Could you check a few things on this drawing? It's one solid part, dimensions in mm from its lowest x, y, z. A direction names the side the tool comes from. Coordinates: 2 decimals unless noted, no trailing zeros. Write each loop counter-clockwise with the first axis right and the second up, starting at its lowest first coordinate (ties: lowest second). Pieces come first, ordered by that corner, then holes.
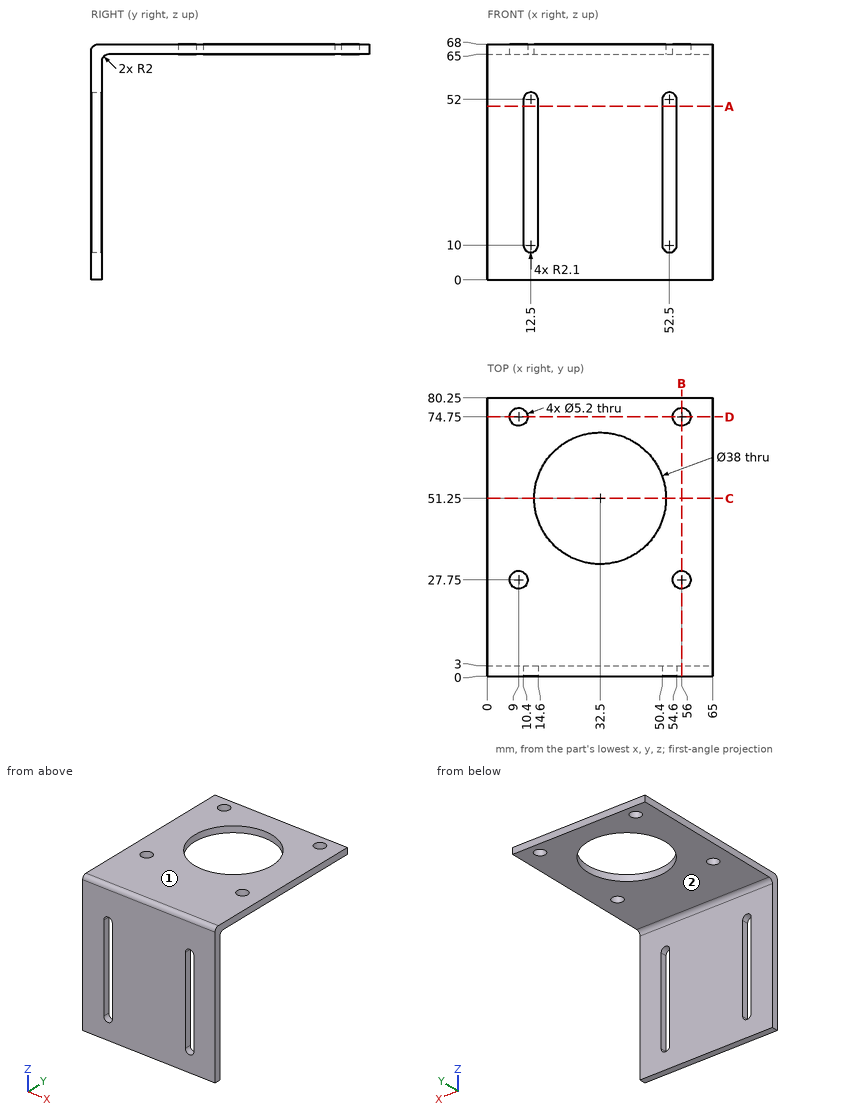
1) Imagine slicing it at D-D on y = 74.75. Please give me the cut outline in (x, z).
Values follow:
outline: (0, 65) - (6.4, 65) - (6.4, 68) - (0, 68) - close; (11.6, 65) - (53.4, 65) - (53.4, 68) - (11.6, 68) - close; (58.6, 65) - (65, 65) - (65, 68) - (58.6, 68) - close
2) Imagine slicing it at B-B on x = 56. Please give me the cut outline in (y, z), then the cut area to 3 significant figures.
Values follow:
outline: (0, 0) - (3, 0) - (3, 63) arc R2 cw to (5, 65) - (25.15, 65) - (25.15, 68) - (2, 68) arc R2 ccw to (0, 66) - close; (30.35, 65) - (72.15, 65) - (72.15, 68) - (30.35, 68) - close; (77.35, 65) - (80.25, 65) - (80.25, 68) - (77.35, 68) - close
area: 405 mm2
3) Will these pins go through, and if not, where does the flat tip stop? pin 1 (8 mm diameter, centred on x = 39.5, z = 9, fed in from +Y); pin 2 (19.5 mm diameter, centred on x = 18, y = 50, fed in from -Z).
Values follow:
pin 1: stops at y = 3
pin 2: stops at z = 65
4) On a 3-axis mill with a long thin cutter (end or side, diameter ignored), from which of +Z, -Z, +X, -X, +Y, -Y can I reach the whole of each face in a straight line? I mean the marked faces 1 and 2. Say none if no direction works.
Values follow:
face 1: +Z, +X, -X, +Y, -Y
face 2: -Z, +X, -X, +Y
5) Imagine slicing it at A-A on z = 50. Please give me the cut outline in (x, y).
Values follow:
outline: (0, 0) - (10.4, 0) - (10.4, 3) - (0, 3) - close; (14.6, 0) - (50.4, 0) - (50.4, 3) - (14.6, 3) - close; (54.6, 0) - (65, 0) - (65, 3) - (54.6, 3) - close
6) Imagine slicing it at C-C on y = 51.25. Please give me the cut outline in (x, z).
Values follow:
outline: (0, 65) - (13.5, 65) - (13.5, 68) - (0, 68) - close; (51.5, 65) - (65, 65) - (65, 68) - (51.5, 68) - close
7) I need wall thicknesses on probe 1 along Y at (x, z) = (26.5, 48); probe 2 along Z at (x, y) = (43, 14.5); probe 3 along Y at (x, z) = (9, 67). Which ranges of each line are inside material? Lowest first, please.
Values follow:
probe 1: y = 0 to 3
probe 2: z = 65 to 68
probe 3: y = 0.27 to 25.15, 30.35 to 72.15, 77.35 to 80.25
